```python
from build123d import *

# Parameters (mm, degrees)
SKETCH1_W           = 92.2
SKETCH1_H           = 49.4
SKETCH1_R           = 1.5
SKETCH1_R_2         = 8.262166988
SKETCH1_R_3         = 8.192856998
SKETCH1_R_4         = 4.886635654
SKETCH1_R_5         = 4.866362118
SKETCH1_R_6         = 5.289603921
SKETCH1_R_7         = 5.006266963
SKETCH1_W_2         = 8.178065913
SKETCH1_H_2         = 16.173235784
SKETCH1_W_3         = 15.980396505
SKETCH1_H_3         = 7.959466721
SKETCH1_W_4         = 7.911671113
SKETCH1_H_4         = 15.979493629
SKETCH1_W_5         = 15.177608392
SKETCH1_H_5         = 9.83005725
BOSS_EXTRUDE1_DEPTH = 2
SKETCH3_W           = 8.178065913
SKETCH3_H           = 16.173235784
SKETCH3_W_2         = 15.980396505
SKETCH3_H_2         = 7.959466721
SKETCH3_W_3         = 7.911671113
SKETCH3_H_3         = 15.979493629
BOSS_EXTRUDE2_DEPTH = 10
SKETCH4_R           = 8.192856998
SKETCH4_R_2         = 8.262166988
SKETCH4_R_3         = 4.886635654
SKETCH4_R_4         = 4.866362118
SKETCH4_R_5         = 5.289603921
SKETCH4_R_6         = 5.006266963
BOSS_EXTRUDE3_DEPTH = 22
SKETCH5_W           = 15.177608392
SKETCH5_H           = 9.83005725
BOSS_EXTRUDE4_DEPTH = 23
SKETCH6_R           = 3.5
BOSS_EXTRUDE5_DEPTH = 20


with BuildPart() as part:
    # Sketch1 → Boss-Extrude1 (new body)
    with BuildSketch(Plane(origin=(0, 0, 0), x_dir=(1, 0, 0), z_dir=(0, 1, 0))):
        with Locations((46.1, 24.7)):
            Rectangle(SKETCH1_W, SKETCH1_H)
        with Locations(Location((3.173958683, 3.331705549, 0), (0, 0, 270))):
            Circle(SKETCH1_R, mode=Mode.SUBTRACT)
        with Locations(Location((88.799397051, 46.406009575, 0), (0, 0, 270))):
            Circle(SKETCH1_R, mode=Mode.SUBTRACT)
        with Locations(Location((88.799397051, 3.331705549, 0), (0, 0, 270))):
            Circle(SKETCH1_R, mode=Mode.SUBTRACT)
        with Locations(Location((21.794183192, 9.960470024, 0), (0, 0, 270))):
            Circle(SKETCH1_R_2, mode=Mode.SUBTRACT)
        with Locations(Location((21.794183192, 28.264813263, 0), (0, 0, 270))):
            Circle(SKETCH1_R_3, mode=Mode.SUBTRACT)
        with Locations(Location((6.541955346, 43.259679485, 0), (0, 0, 270))):
            Circle(SKETCH1_R_4, mode=Mode.SUBTRACT)
        with Locations(Location((17.408846233, 43.259679485, 0), (0, 0, 270))):
            Circle(SKETCH1_R_5, mode=Mode.SUBTRACT)
        with Locations(Location((28.27573712, 43.259679485, 0), (0, 0, 270))):
            Circle(SKETCH1_R_6, mode=Mode.SUBTRACT)
        with Locations(Location((39.303222454, 43.259679485, 0), (0, 0, 270))):
            Circle(SKETCH1_R_7, mode=Mode.SUBTRACT)
        with Locations((6.70046548, 15.533525735)):
            Rectangle(SKETCH1_W_2, SKETCH1_H_2, mode=Mode.SUBTRACT)
        with Locations((59.680344983, 44.042689104)):
            Rectangle(SKETCH1_W_3, SKETCH1_H_3, mode=Mode.SUBTRACT)
        with Locations((86.603660988, 25.480585451)):
            Rectangle(SKETCH1_W_4, SKETCH1_H_4, mode=Mode.SUBTRACT)
        with Locations((74.28567685, 6.953513815)):
            Rectangle(SKETCH1_W_5, SKETCH1_H_5, mode=Mode.SUBTRACT)
    extrude(amount=BOSS_EXTRUDE1_DEPTH)

    # Sketch3 → Boss-Extrude2 (add)
    with BuildSketch(Plane(origin=(0, 0, 0), x_dir=(-1, 0, 0), z_dir=(0, -1, 0))):
        with Locations((-6.70046548, 15.533525735)):
            Rectangle(SKETCH3_W, SKETCH3_H)
        with Locations((-59.680344983, 44.042689104)):
            Rectangle(SKETCH3_W_2, SKETCH3_H_2)
        with Locations((-86.603660988, 25.480585451)):
            Rectangle(SKETCH3_W_3, SKETCH3_H_3)
    extrude(amount=-BOSS_EXTRUDE2_DEPTH)

    # Sketch4 → Boss-Extrude3 (add)
    with BuildSketch(Plane(origin=(0, 0, 0), x_dir=(-1, 0, 0), z_dir=(0, -1, 0))):
        with Locations(Location((-21.794183192, 28.264813263, 0), (0, 0, 90))):
            Circle(SKETCH4_R)
        with Locations(Location((-21.794183192, 9.960470024, 0), (0, 0, 90))):
            Circle(SKETCH4_R_2)
        with Locations(Location((-6.541955346, 43.259679485, 0), (0, 0, 90))):
            Circle(SKETCH4_R_3)
        with Locations(Location((-17.408846233, 43.259679485, 0), (0, 0, 90))):
            Circle(SKETCH4_R_4)
        with Locations(Location((-28.27573712, 43.259679485, 0), (0, 0, 90))):
            Circle(SKETCH4_R_5)
        with Locations(Location((-39.303222454, 43.259679485, 0), (0, 0, 90))):
            Circle(SKETCH4_R_6)
    extrude(amount=-BOSS_EXTRUDE3_DEPTH)

    # Sketch5 → Boss-Extrude4 (add)
    with BuildSketch(Plane(origin=(0, 0, 0), x_dir=(-1, 0, 0), z_dir=(0, -1, 0))):
        with Locations((-74.28567685, 6.953513815)):
            Rectangle(SKETCH5_W, SKETCH5_H)
    extrude(amount=-BOSS_EXTRUDE4_DEPTH)

    # Sketch6 → Boss-Extrude5 (add)
    with BuildSketch(Plane.XY.offset(-2.03848519)):
        with Locations((74.28567685, 15)):
            Circle(SKETCH6_R)
    extrude(amount=BOSS_EXTRUDE5_DEPTH)


solid = part.part
```
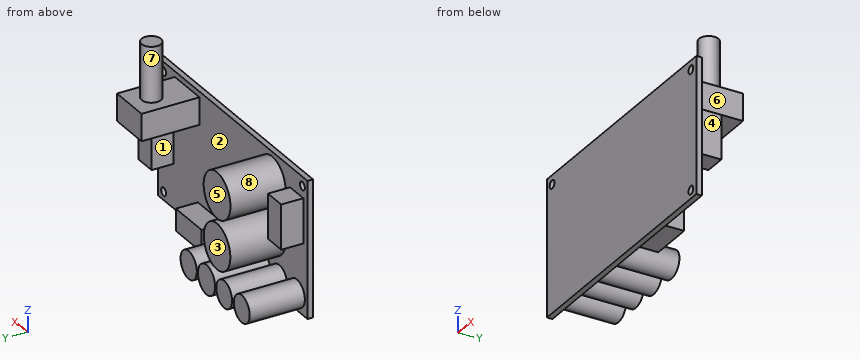
Geometry: final body of the model. Coordinates: model frame, mm. Face numbers are marked on the shaded views. A direction names the side the tool comes from. Round coordinates to 2 decimals unless told otherwise and drop trailing zeros. Loops run counter-clockwise (first coordinate to the right, second up) from the corner with the lowest first, then second, coordinate; pieces in that order, holes last.
Item 1: Contact query for flat-ended pins moving along their axis: P1, Ø4, axis at y = 4.5, z = -43, coming from the +X side; P2, Ø3, axis at x = 37, z = -42, coming from the +Y side; P3, Ø5, axis at x = 78, z = -15.5, coming from the +Y side. Output: stop coordinate, or through.
Checked values:
P1: stops at x = 67.67
P2: stops at y = 22
P3: stops at y = 2
Item 2: Section B-B, the plane x = 60. Output: boundary loops of the cut face in (y, z), plus the area to 3 significant figures.
Checked values:
outline: (0, -49.4) - (2, -49.4) - (2, -48.02) - (10, -48.02) - (10, -40.06) - (2, -40.06) - (2, 0) - (0, 0) - close
area: 162 mm2
Item 3: Section A-A, the plane y = 15. Output: boundary loops of the cut face in (x, z).
Checked values:
outline: circle Ø9.77 at (6.54, -43.26); circle Ø9.73 at (17.41, -43.26); circle Ø16.52 at (21.79, -9.96); circle Ø16.39 at (21.79, -28.26); circle Ø10.58 at (28.28, -43.26); circle Ø10.01 at (39.3, -43.26); (66.7, -11.87) - (81.87, -11.87) - (81.87, -2.04) - (77.79, -2.04) - (77.79, 17.96) - (70.79, 17.96) - (70.79, -2.04) - (66.7, -2.04) - close
Item 4: Section C-C, the plane y = 6.75. State how many separate pieces and enclosed holes the cut face has, plus the area to 3 significant figures.
Checked values:
separate pieces: 10
enclosed holes: 0
area: 1,280 mm2
Item 5: Section D-D, the plane z = 8. Output: boundary loops of the cut face in (x, y).
Checked values:
outline: circle Ø7 at (74.29, 15)
Item 6: Mould query, pull axis X, two halves, no side actions, for the marked faces 1, 2, 3 and 4. Classes: released by +X, released by -X, zero draft, split by the parting line, or undercut.
Checked values:
face 1: undercut
face 2: undercut
face 3: zero draft
face 4: released by +X
Item 7: Reachability of the marked faces 5, 6, 7 and 8 from +Z, -Z, +X, -X, +Y, -Y: full face, straight path, thin tool, end or side. Return the list, or none.
Checked values:
face 5: +Z, -Z, -X, +Y
face 6: +Z, -Z, +X, +Y
face 7: +Z
face 8: +Y
Item 8: Line query: L1, parallel to Z at x = 7, y = 9.5; L2, parallel to Z at x = 14.5, y = 21.5; L3, parallel to X at y = 20, z = -45. Output: solid intervals per line, ascending.
Checked values:
L1: z = -48.12 to -38.39, -23.62 to -7.45
L2: z = -47.16 to -39.36, -32 to -24.53, -13.84 to -6.08
L3: x = 1.98 to 11.11, 12.86 to 21.95, 23.28 to 33.27, 34.61 to 44
